from build123d import *

# Parameters (mm, degrees)
SKETCH_1_W          = 38.6
SKETCH_1_H          = 24
EXTRUDE_1_DEPTH     = 9.7
SKETCH_2_W          = 0.75
SKETCH_2_H          = 21
EXTRUDE_2_DEPTH     = 4
CHAMFER_1_SIZE      = 3
SKETCH_3_W          = 4
SKETCH_3_H          = 7.3
CUT_EXTRUDE_1_DEPTH = 6.2
SKETCH_4_R          = 2.5
CUT_EXTRUDE_2_DEPTH = 4.5


with BuildPart() as part:
    # 草图1 → 凸台-拉伸1 (new body)
    with BuildSketch(Plane(origin=(28.693608134, -23.996349429, -44.112502039), x_dir=(1, 0, 0), z_dir=(0, 0, 1))):
        with Locations((-46.492248891, -33.863193326)):
            Rectangle(SKETCH_1_W, SKETCH_1_H)
    extrude(amount=EXTRUDE_1_DEPTH)

    # 草图2 → 凸台-拉伸2 (add)
    with BuildSketch(Plane.ZY.offset(37.098640757)):
        with Locations((-42.737502039, -57.859542755)):
            Rectangle(SKETCH_2_W, SKETCH_2_H)
    extrude(amount=EXTRUDE_2_DEPTH)

    # 倒角1
    chamfer_1_edges = [part.edges().sort_by_distance(p)[0] for p in [
        (1.501359243, -57.859542755, -34.412502039),
    ]]
    chamfer(chamfer_1_edges, length=CHAMFER_1_SIZE)

    # 草图3 → 切除-拉伸1 (cut)
    with BuildSketch(Plane.XY.offset(-34.412502039)):
        with Locations((-0.498640757, -57.859542755)):
            Rectangle(SKETCH_3_W, SKETCH_3_H)
    extrude(amount=-CUT_EXTRUDE_1_DEPTH, mode=Mode.SUBTRACT)

    # 草图4 → 切除-拉伸2 (cut, through all)
    with BuildSketch(Plane.XY.offset(-40.612502039)):
        with Locations((1.501359243, -57.859542755)):
            Circle(SKETCH_4_R)
    extrude(amount=-CUT_EXTRUDE_2_DEPTH, mode=Mode.SUBTRACT)


solid = part.part
Source: CAD feature listing. Evaluate the final solid. Frame: model axes, mm. A direction names the side the tool comes from. Round coordinates to 2 decimals unless told otherwise and drop trailing zeros. Order: outer loops, then holes, each group sorted by start corner. A loop starts at its lowest first (then second) coordinate and runs counter-clockwise, first axis right, second up. Notation, with made-up numbers: (-1.5, -12.75) - (34.5, -12.75) arc R20 ccw to (34.5, 23.25) - close; hole circle Ø6 at (43.25, 30.25). An arc over 180 degrees is marked (long way). Use a Markdown table: item, result. Add a question column.
1. Set-up query: faces 5 (the flat face through (-18, -58, -44.113)), 6 (the flat face through (-2.499, -58, -37)), 7 (the flat face through (0.02, -65.74, -35.93)), 8 (the flat face through (-39, -58, -42.363)), 9 (the flat face through (-39, -58, -43.113)). Return all of +Z, -Z, +X, -X, +Y, -Y with unobstructed straight access to the full face (end or side cutting, diameter ignored); none if empty.
2. First-contact query: pin 1 (0.6 mm diameter, centred on x = -40, z = -42.5, fed in from +Y); pin 2 (4.5 mm diameter, centred on x = -40, y = -53, fed in from +Z); pin 3 (2 mm diameter, centred on x = -40, y = -59.5, fed in from -Z). Flat tips, straight axial feed; report the tip coordinate or a pass-through.
3. Section query B-B (z = -39.25). Return the cut outline in (x, y), then the cut area to 3 significant figures.
4. Section query A-A (y = -53.75). Return the cut outline in (x, z).
5. Section query D-D (z = -41.75). Return the cut outline in (x, y).
6. Section query C-C (y = -56.75). Return the cut outline in (x, z).
7. Line query: probe 1 along Y at (x, z) = (0, -40); probe 2 along Z at (x, y) = (-39, -57); probe 3 along Z at (x, y) = (-1, -58.25). Output: solid intervals per line, ascending.
8. Mould query, pull axis Y, two halves, no side actions, for faces 1 (the flat face through (-18, -45.86, -39)), 2 (the flat face through (-1, -54.21, -38)), 3 (the cylindrical face through (-0.998, -57.805, -42.338)), 4 (the flat face through (0.02, -50.09, -35.93)). Classes: +Y half, -Y half, draft (parallel to the pull), parting line (faces both ways), or undercut.
Derived:
| question | item | result |
|---|---|---|
| 1 | face 5 | -Z, +X, -X, +Y, -Y |
| 1 | face 6 | +Z, +X |
| 1 | face 7 | +Z, +X, +Y, -Y |
| 1 | face 8 | +Z, -X, +Y, -Y |
| 1 | face 9 | -Z, -X, +Y, -Y |
| 2 | pin 1 | y = -47.36 |
| 2 | pin 2 | z = -42.36 |
| 2 | pin 3 | z = -43.11 |
| 3 | outline | (-37.1, -69.86) - (1.5, -69.86) - (1.5, -61.51) - (-2.5, -61.51) - (-2.5, -54.21) - (1.5, -54.21) - (1.5, -45.86) - (-37.1, -45.86) - close |
| 3 | area | 897 mm2 |
| 4 | outline | (-41.1, -43.11) - (-37.1, -43.11) - (-37.1, -44.11) - (1.5, -44.11) - (1.5, -37.41) - (-1.5, -34.41) - (-37.1, -34.41) - (-37.1, -42.36) - (-41.1, -42.36) - close |
| 5 | outline | (-37.1, -69.86) - (1.5, -69.86) - (1.5, -60.36) arc R2.5 cw to (1.5, -55.36) - (1.5, -45.86) - (-37.1, -45.86) - close |
| 6 | outline | (-41.1, -43.11) - (-37.1, -43.11) - (-37.1, -44.11) - (-0.74, -44.11) - (-0.74, -40.61) - (-2.5, -40.61) - (-2.5, -34.41) - (-37.1, -34.41) - (-37.1, -42.36) - (-41.1, -42.36) - close |
| 7 | probe 1 | -69.86 to -61.51, -54.21 to -45.86 |
| 7 | probe 2 | -43.11 to -42.36 |
| 7 | probe 3 | -44.11 to -40.61 |
| 8 | face 1 | +Y half |
| 8 | face 2 | undercut |
| 8 | face 3 | undercut |
| 8 | face 4 | draft |
